from build123d import *

# Parameters (mm, degrees)
EXTRUDE1_DEPTH     = 2.286
SKETCH2_R          = 2.413
CUT_EXTRUDE1_DEPTH = 3.286
LPATTERN1_COUNT    = 9
LPATTERN1_PITCH    = 12.7


with BuildPart() as part:
    # Sketch1 → Extrude1 (new body)
    with BuildSketch(Plane.XY):
        with BuildLine():
            Line((-50.8, -6.35), (50.8, -6.35))
            ThreePointArc((50.8, -6.35), (57.15, 0), (50.8, 6.35))
            Line((50.8, 6.35), (-50.8, 6.35))
            ThreePointArc((-50.8, 6.35), (-57.15, 0), (-50.8, -6.35))
        make_face()
    extrude(amount=EXTRUDE1_DEPTH)

    # Sketch2 → Cut-Extrude1 (cut, through all)
    with BuildSketch(Plane.XY.offset(2.286)):
        with Locations((-50.8, 0)):
            Circle(SKETCH2_R)
    cut_extrude1 = extrude(amount=-CUT_EXTRUDE1_DEPTH, mode=Mode.SUBTRACT)

    # LPattern1: Cut-Extrude1 ×9
    with Locations(*[(i * LPATTERN1_PITCH, 0, 0) for i in range(1, LPATTERN1_COUNT)]):
        add(cut_extrude1, mode=Mode.SUBTRACT)


solid = part.part
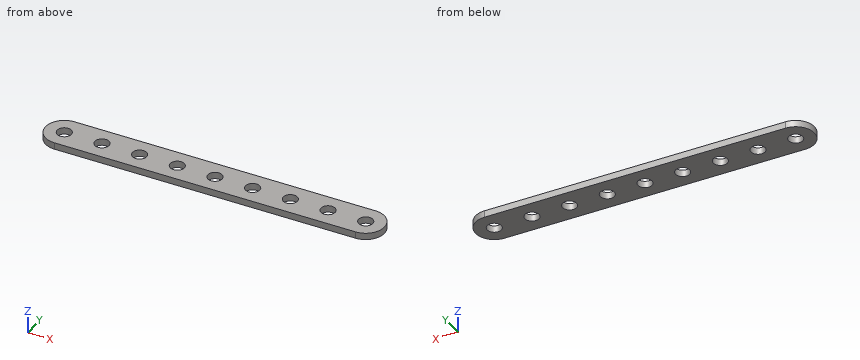
Model file for the job. Use its own axes, mm. Coordinates: 2 decimals unless noted, no trailing zeros. Order: outer loops, then holes, each group sorted by start corner. A loop starts at its lowest first (then second) coordinate and runs counter-clockwise, first axis right, second up. Notation, with made-up numbers: M 19.5,74.25 L 63.5,74.25 A21 ccw 63.5,111.25 Z; hole C -2,20.5 d7. An arc over 180 degrees is marked long. Return JSON: item names as keys, results as strings.
1. Saw through at A-A (x = -25.4). Give the cut face in (y, z), and give its area (3 significant figures).
Ans:
{"outline": "M -6.35,0 L -2.41,0 L -2.41,2.29 L -6.35,2.29 Z; M 2.41,0 L 6.35,0 L 6.35,2.29 L 2.41,2.29 Z", "area": "18.0 mm^2"}
2. Drill centre lines: probe 1 along Y at (x, z) = (0, 1.1); probe 2 along X at (y, z) = (-5.5, 0.95). Where is each one in solid material? Low to high.
Ans:
{"probe 1": "-6.35 to -2.41, 2.41 to 6.35", "probe 2": "-53.97 to 53.97"}
3. Saw through at D-D (x = 14). Give the cut face in (y, z), and give its area (3 significant figures).
Ans:
{"outline": "M -6.35,0 L -2.03,0 L -2.03,2.29 L -6.35,2.29 Z; M 2.03,0 L 6.35,0 L 6.35,2.29 L 2.03,2.29 Z", "area": "19.7 mm^2"}
4. Flat gauge pins, fed straight in: pin 1 (4.5 mm diameter, centred on x = 0, y = 0, fed in from -Z); pin 2 (1 mm diameter, centred on y = -5, z = 0.5, fed in from +X); pin 3 (1 mm diameter, centred on y = -4, z = 1, fed in from -X). Where does each tip first touch, or does it go through?
Ans:
{"pin 1": "through", "pin 2": "x = 55.28", "pin 3": "x = -56.1"}
5. Saw through at B-B (z = 0.7). Give the number of separate pieces and of enclosed holes in the cut face, and give its area (3 significant figures).
Ans:
{"separate pieces": "1", "enclosed holes": "9", "area": "1,250 mm^2"}
